Source: three-view drawing plus pictorial views. Frame: mm from the lowest corner of the part. Give positions to 0.01 mm unless a question says otherwise; leave off trailing zeros. Loops run counter-clockwise (first coordinate to the right, second up) from the corner with the lowest first, then second, coordinate; pieces in that order, holes last. Notation, with made-up numbers: (72, 59) - (105, 59) arc R29 cw to (105, 81) - close; hole circle Ø1 at (87.25, -25). An arc over 180 degrees is marked (long way). One line per item, written item: value.
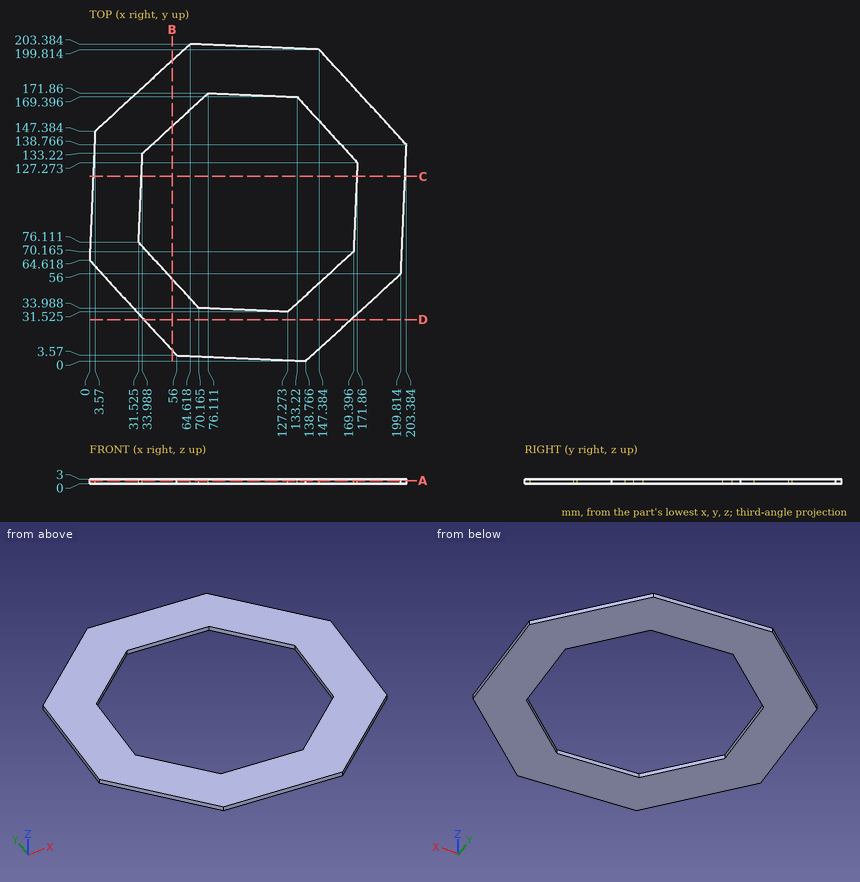
Item 1: Section B-B, the plane x = 53. Output: boundary loops of the cut face in (y, z).
Verdict:
outline: (6.84, 0) - (52.7, 0) - (52.7, 3) - (6.84, 3) - close; (150.66, 0) - (192.73, 0) - (192.73, 3) - (150.66, 3) - close
Item 2: Section C-C, the plane y = 118.5. Output: boundary loops of the cut face in (x, z).
Verdict:
outline: (2.32, 0) - (33.35, 0) - (33.35, 3) - (2.32, 3) - close; (171.48, 0) - (202.51, 0) - (202.51, 3) - (171.48, 3) - close
Item 3: Material intervals for L1, parallel to Y at x = 131, z = 0.4 (1 decimal); L2, parallel to X at y = 66, z = 2.95 (1 decimal); L3, parallel to X at y = 147, z = 1.05 (1 decimal), sorted ascending.
Verdict:
L1: y = 0.3 to 34.9, 169.5 to 200.5
L2: x = 0.1 to 40.8, 164.9 to 200.2
L3: x = 3.6 to 49, 153.8 to 195.8
Item 4: Section A-A, the plane z = 1.95. Output: boundary loops of the cut face in (x, y) (1 decimal), and give its area (3 significant figures).
Verdict:
outline: (0, 64.6) - (56, 3.6) - (138.8, 0) - (199.8, 56) - (203.4, 138.8) - (147.4, 199.8) - (64.6, 203.4) - (3.6, 147.4) - close; hole (31.5, 76.1) - (70.2, 34) - (127.3, 31.5) - (169.4, 70.2) - (171.9, 127.3) - (133.2, 169.4) - (76.1, 171.9) - (34, 133.2) - close
area: 17,400 mm^2
Item 5: Pin query (flat end, axial travel): P1, Ø1.5, axis at y = 75, z = 0.5, coming from the +X side; P2, Ø1.5, axis at x = 104.5, z = 1.5, coming from the -Y side (1 decimal); P3, Ø1.5, axis at y = 105, z = 1, coming from the +X side. Return the tip coordinate at first contact, or that it passes through.
Verdict:
P1: stops at x = 200.67
P2: stops at y = 1.4
P3: stops at x = 201.96
Item 6: Section D-D, the plane y = 26.5. Output: boundary loops of the cut face in (x, z) (1 decimal), and give its area (3 significant figures).
Verdict:
outline: (35, 0) - (167.7, 0) - (167.7, 3) - (35, 3) - close
area: 398 mm^2
